```python
from build123d import *

# Parameters (mm, degrees)
SKETCH1_R           = 2.1
SKETCH1_R_2         = 2.25
SKETCH1_R_3         = 1.5
BOSS_EXTRUDE2_DEPTH = 3


with BuildPart() as part:
    # Sketch1 → Boss-Extrude2 (new body)
    with BuildSketch(Plane.XY):
        with BuildLine():
            Line((-27.248541099, 19.686096161), (-57.707535143, 4.573632695))
            Line((-57.707535143, 4.573632695), (-57.707535143, -17.510368624))
            Line((-57.707535143, -17.510368624), (-15.340272848, -16.957179715))
            Line((-15.340272848, -16.957179715), (-21.390839368, 17.496417988))
            ThreePointArc((-21.390839368, 17.496417988), (-23.801885744, 19.97645801), (-27.248541099, 19.686096161))
        make_face()
        with Locations((-38.131817883, -9.421553771)):
            Circle(SKETCH1_R, mode=Mode.SUBTRACT)
        with Locations((-25.381817883, 15.923737268)):
            Circle(SKETCH1_R_2, mode=Mode.SUBTRACT)
        with Locations((-23.071502026, -4.400056763)):
            Circle(SKETCH1_R_3, mode=Mode.SUBTRACT)
        with Locations((-50.787681668, -9.435461189)):
            Circle(SKETCH1_R_3, mode=Mode.SUBTRACT)
    extrude(amount=BOSS_EXTRUDE2_DEPTH)


solid = part.part
```
Check sheet for the modelled part. Datum: model origin and axes. Units: mm. Round coordinates to 2 decimals unless told otherwise and drop trailing zeros. Loops run counter-clockwise (first coordinate to the right, second up) from the corner with the lowest first, then second, coordinate; pieces in that order, holes last. Notation, with made-up numbers: (78, -23.75) - (106, -23.75) arc R9 ccw to (106, -14.75) - close; hole circle Ø2 at (85, 80.5). An arc over 180 degrees is marked (long way). Answer as a JSON object with one key per item and string values. Group by question number.
Q1. Mould release check, pull along Y, two halves, no side actions. Record for faces 1 (the face through (-57.708, -6, 1)), 2 (the face through (-51.89, -8.42, 1.48)), 3 (the face through (-18.323, 0.028, 1.479)): released by +Y, released by -Y, zero draft, split by the parting line, or undercut.
Q2. Scan lines: line 1 along Y through (x, z) = (-25.5, 1.3); line 2 along Y through (x, z) = (-22.5, 1.8); line 3 along Y through (x, z) = (-47.5, 1.4). Record each from-to range of solid material in increasing order. Write a range as [from, to].
Q3. Sectioned sample at C-C, the plane y = 16.5. Enter the section's corners in (x, z), plus the area to 3 significant figures.
Q4. Sectioned sample at D-D, the plane y = -8.5. Enter the section's corners in (x, z), plus the area to 3 significant figures.
Q5. Sectioned sample at A-A, the plane x = -26. Enter the section's corners in (y, z).
Q6. Sectioned sample at B-B, the plane z = 0.7. Enter the section's corners in (x, y).
Solution:
{
 "1": {"face 1": "zero draft", "face 2": "undercut", "face 3": "released by +Y"},
 "2": {"line 1": "y = [-17.09, 13.68], [18.17, 20.22]", "line 2": "y = [-17.05, -5.79], [-3.01, 19.18]", "line 3": "y = [-17.38, 9.64]"},
 "3": {"outline": "(-33.67, 0) - (-27.56, 0) - (-27.56, 3) - (-33.67, 3) - close; (-23.21, 0) - (-21.22, 0) - (-21.22, 3) - (-23.21, 3) - close", "area": "24.3 mm²"},
 "4": {"outline": "(-57.71, 0) - (-51.96, 0) - (-51.96, 3) - (-57.71, 3) - close; (-49.62, 0) - (-40.02, 0) - (-40.02, 3) - (-49.62, 3) - close; (-36.24, 0) - (-16.83, 0) - (-16.83, 3) - (-36.24, 3) - close", "area": "104 mm²"},
 "5": {"outline": "(-17.1, 0) - (13.76, 0) - (13.76, 3) - (-17.1, 3) - close; (18.09, 0) - (20.16, 0) - (20.16, 3) - (18.09, 3) - close"},
 "6": {"outline": "(-57.71, -17.51) - (-15.34, -16.96) - (-21.39, 17.5) arc R4.05 ccw to (-27.25, 19.69) - (-57.71, 4.57) - close; hole circle Ø3 at (-50.79, -9.44); hole circle Ø4.2 at (-38.13, -9.42); hole circle Ø4.5 at (-25.38, 15.92); hole circle Ø3 at (-23.07, -4.4)"}
}
